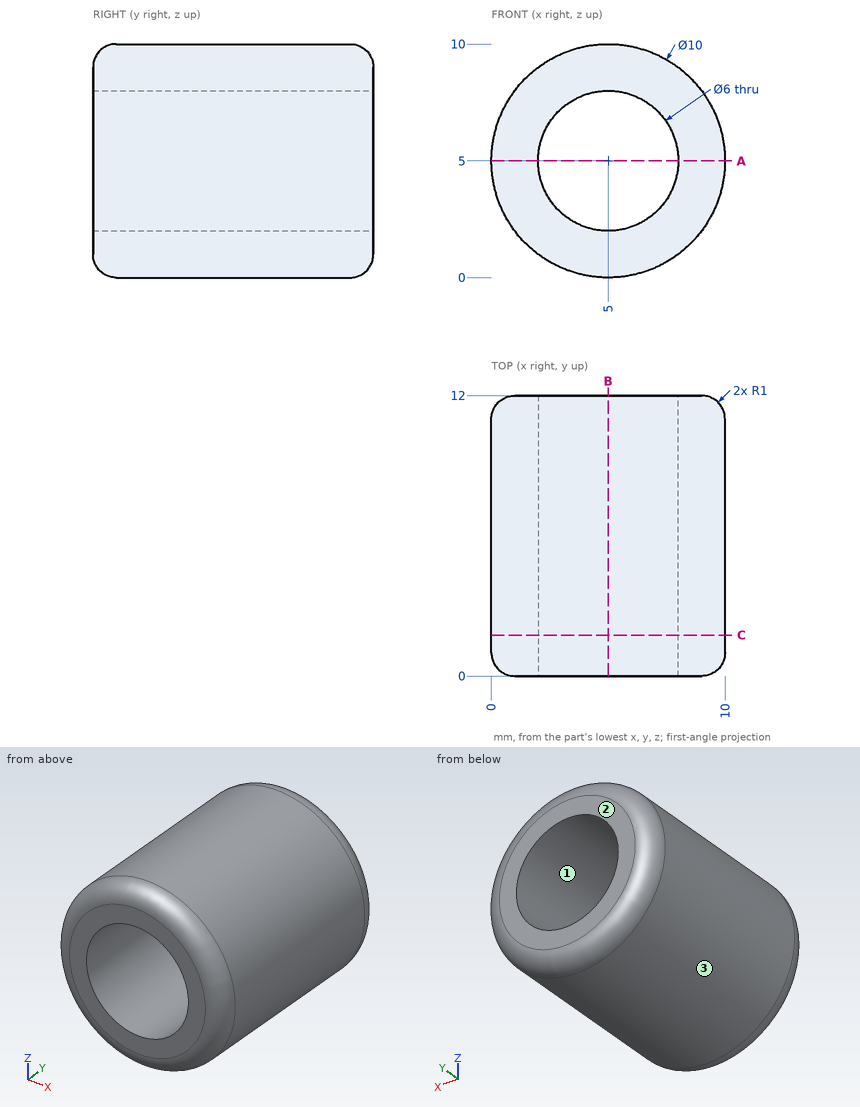
Study the drawing (mm; zero at the part's minimum x, y, z) and answer. Coordinates: 2 decimals unless noted, no trailing zeros. Loops run counter-clockwise (first coordinate to the right, second up) from the corner with the lowest first, then second, coordinate; pieces in that order, holes last. Notation, with made-up numbers: (-5.5, 76.25) -> (26.5, 76.25) arc R16 cw to (26.5, 103.25) -> close; hole circle Ø11 at (-27.5, 85.5). An arc over 180 degrees is marked (long way). Answer in a Markdown table with one row per item. Add a question column.
1. A flat-ended cylindrical pin translates along its axis: P1, Ø2, axis at y = 2.5, z = 1.5, coming from the +X side. Find the tip coordinate at first contact, or state that the pin passes through.
2. The part is cut by section A-A, the plane z = 5. Write down the section's boundary in (x, y).
3. The part is cut by section B-B, the plane x = 5. Write down the section's boundary in (y, z).
4. The part is cut by section C-C, the plane y = 1.75. Write down the section's boundary in (x, z), then the cut area to 3 significant figures.
5. Determine the mould class of the marked faces 1, 2 and 3 for opening direction X: +X half, -X half, draft (parallel to the pull), parting line (faces both ways), or undercut.
6. Consider line 1 (Z direction, x = 5, y = 2.5); line 2 (Z direction, x = 9, y = 10); line 3 (X direction, y = 11.75, z = 7.75). Determine where each line is inside the solid, lowest interval first. Write a range as [from, to].
Answer below:
| question | item | result |
|---|---|---|
| 1 | P1 | x = 9.33 |
| 2 | outline | (0, 1) arc R1 ccw to (1, 0) -> (2, 0) -> (2, 12) -> (1, 12) arc R1 ccw to (0, 11) -> close; (8, 0) -> (9, 0) arc R1 ccw to (10, 1) -> (10, 11) arc R1 ccw to (9, 12) -> (8, 12) -> close |
| 3 | outline | (0, 1) arc R1 ccw to (1, 0) -> (11, 0) arc R1 ccw to (12, 1) -> (12, 2) -> (0, 2) -> close; (0, 8) -> (12, 8) -> (12, 9) arc R1 ccw to (11, 10) -> (1, 10) arc R1 ccw to (0, 9) -> close |
| 4 | outline | circle Ø10 at (5, 5); hole circle Ø6 at (5, 5) |
| 4 | area | 50.3 mm2 |
| 5 | face 1 | undercut |
| 5 | face 2 | draft |
| 5 | face 3 | parting line |
| 6 | line 1 | [0, 2], [8, 10] |
| 6 | line 2 | [2, 8] |
| 6 | line 3 | [1.24, 3.8], [6.2, 8.76] |
